from build123d import *

# Parameters (mm, degrees)
SKETCH_1_W          = 80
SKETCH_1_H          = 80
EXTRUDE_1_DEPTH     = 6
SKETCH_2_R          = 1
CUT_EXTRUDE_1_DEPTH = 57.885850613
SKETCH_3_W          = 80
SKETCH_3_H          = 6
EXTRUDE_2_DEPTH     = 80
SKETCH_4_W          = 56
SKETCH_4_H          = 35
EXTRUDE_3_DEPTH     = 28
SKETCH_5_W          = 48
SKETCH_5_H          = 24
CUT_EXTRUDE_2_DEPTH = 31


with BuildPart() as part:
    # ｽｹｯﾁ1 → ﾎﾞｽ - 押し出し1 (new body)
    with BuildSketch(Plane(origin=(0, 0, 0), x_dir=(1, 0, 0), z_dir=(0, 1, 0))):
        Rectangle(SKETCH_1_W, SKETCH_1_H)
    extrude_1 = extrude(amount=EXTRUDE_1_DEPTH)

    # ｽｹｯﾁ2 → ｶｯﾄ - 押し出し1 (cut, through all)
    with BuildSketch(Plane(origin=(0, 6, 0), x_dir=(1, 0, 0), z_dir=(0, 1, 0))):
        with Locations(Location((-10.5, 10.5, 0), (0, 0, 270))):
            Circle(SKETCH_2_R)
        with Locations(Location((10.5, 10.5, 0), (0, 0, 270))):
            Circle(SKETCH_2_R)
        with Locations(Location((10.5, -10.5, 0), (0, 0, 270))):
            Circle(SKETCH_2_R)
        with Locations(Location((-10.5, -10.5, 0), (0, 0, 270))):
            Circle(SKETCH_2_R)
    cut_extrude_1 = extrude(amount=-CUT_EXTRUDE_1_DEPTH, mode=Mode.SUBTRACT)

    # ﾐﾗｰ9: ﾎﾞｽ - 押し出し1, ｶｯﾄ - 押し出し1 across plane
    add(extrude_1.mirror(Plane(origin=(40, 6, -40), x_dir=(0, 0, 1), z_dir=(-1, 0, 0))))
    add(cut_extrude_1.mirror(Plane(origin=(40, 6, -40), x_dir=(0, 0, 1), z_dir=(-1, 0, 0))), mode=Mode.SUBTRACT)

    # ﾐﾗｰ10: ﾎﾞｽ - 押し出し1 across plane
    add(extrude_1.mirror(Plane(origin=(-40, 6, 40), x_dir=(1, 0, 0), z_dir=(0, 0, -1))))

    # ｽｹｯﾁ3 → ﾎﾞｽ - 押し出し2 (add)
    with BuildSketch(Plane(origin=(40, 0, 0), x_dir=(0, 0, -1), z_dir=(1, 0, 0))):
        with Locations((-80, 3)):
            Rectangle(SKETCH_3_W, SKETCH_3_H)
    extrude(amount=EXTRUDE_2_DEPTH)

    # ｽｹｯﾁ4 → ﾎﾞｽ - 押し出し3 (add)
    with BuildSketch(Plane(origin=(0, 6, 0), x_dir=(1, 0, 0), z_dir=(0, 1, 0))):
        with Locations((0, -86.5)):
            Rectangle(SKETCH_4_W, SKETCH_4_H)
    extrude(amount=EXTRUDE_3_DEPTH)

    # ｽｹｯﾁ5 → ｶｯﾄ - 押し出し2 (cut)
    with BuildSketch(Plane(origin=(0, 0, 69), x_dir=(-1, 0, 0), z_dir=(0, 0, -1))):
        with Locations((0, 18)):
            Rectangle(SKETCH_5_W, SKETCH_5_H)
    extrude(amount=-CUT_EXTRUDE_2_DEPTH, mode=Mode.SUBTRACT)


solid = part.part
Check sheet for the modelled part. Datum: model origin and axes. Units: mm. A direction names the side the tool comes from. Give positions to 0.01 mm unless a question says otherwise; leave off trailing zeros. Write each loop counter-clockwise with the first axis right and the second up, starting at its lowest first coordinate (ties: lowest second). Pieces come first, ordered by that corner, then holes. Notation, with made-up numbers: (-38, 45.5) -> (6, 45.5) arc R27 ccw to (6, 74.5) -> close; hole circle Ø7 at (64, 32). An arc over 180 degrees is marked (long way). One line per item, written item: value. Start each with the question number.
Item 1: Section check A-A on z = 77.5. Record the cut outline in (x, y).
Item 2: Tool access check on faces 4 (the flat face through (0, 20, 104)), 5 (the flat face through (1.9, 30.3, 69)), 6 (the flat face through (28, 20, 87)). Record the directions out of +Z, -Z, +X, -X, +Y, -Y that give a thin tool (end or side, any length) a straight path to the whole face; none if there is none.
Item 3: Draft check along X on faces 1 (the flat face through (0, 18, 100)), 2 (the flat face through (120, 3, 41)), 3 (the flat face through (41, 3, -40)). Enter one of: +X half, -X half, draft (parallel to the pull), parting line (faces both ways), or undercut.
Item 4: Gauge pin test, flat ends, axial feed: pin 1 (2.5 mm diameter, centred on x = 10.5, z = 10.5, fed in from +Y); pin 2 (7 mm diameter, centred on y = 17.5, z = 87.5, fed in from +X); pin 3 (7 mm diameter, centred on y = 14, z = 86.5, fed in from -X); pin 4 (1.6 mm diameter, centred on x = -10.5, z = 10.5, fed in from -Y). Record the tip position at first contact, or that the pin passes through.
Item 5: Section check D-D on z = -16. Record the cut outline in (x, y), then the cut area to 3 significant figures.
Item 6: Section check B-B on y = 21. Record the cut outline in (x, z), then the cut area to 3 significant figures.
Item 7: Material ranges on probe 1 along X at (y, z) = (1.5, 10.5); probe 2 along Z at (x, y) = (90.5, 4.2); probe 3 along Z at (x, y) = (69, 2), recorded low to high. Write a range as from..to.
Item 8: Section check C-C on x = 105.5. Record the cut outline in (y, z).
Results list:
1. outline: (-40, 0) -> (120, 0) -> (120, 6) -> (28, 6) -> (28, 34) -> (-28, 34) -> (-28, 6) -> (-40, 6) -> close; hole (-24, 6) -> (24, 6) -> (24, 30) -> (-24, 30) -> close
2. face 4: +Z, +X, -X, +Y
2. face 5: -Z, +X, -X, +Y
2. face 6: +Z, -Z, +X, +Y
3. face 1: undercut
3. face 2: +X half
3. face 3: draft
4. pin 1: y = 6
4. pin 2: x = 28
4. pin 3: x = -28
4. pin 4: through
5. outline: (-40, 0) -> (120, 0) -> (120, 6) -> (-40, 6) -> close
5. area: 960 mm²
6. outline: (-28, 69) -> (-24, 69) -> (-24, 100) -> (24, 100) -> (24, 69) -> (28, 69) -> (28, 104) -> (-28, 104) -> close
6. area: 472 mm²
7. probe 1: -40..-11.5, -9.5..9.5, 11.5..68.5, 70.5..89.5, 91.5..120
7. probe 2: -40..-11.5, -9.5..9.5, 11.5..120
7. probe 3: -40..-11.37, -9.63..9.63, 11.37..120
8. outline: (0, -40) -> (6, -40) -> (6, 120) -> (0, 120) -> close
